from build123d import *

# Parameters (mm, degrees)
F0_R     = 17.275
F1_DEPTH = 18
F3_D     = 32
F4_R     = 16.275
F5_DEPTH = 5
F6_R     = 4.99999


# Not quite as in the source:
# - a fillet or chamfer is up to 0.001 mm smaller than in the source, because OpenCascade refuses the exact size


with BuildPart() as f1:
    # F0 (on Front) → F1 (new body)
    with BuildSketch(Plane.XZ):
        Circle(F0_R)
    extrude(amount=F1_DEPTH)

    # F3 (through all)
    with Locations(Plane(origin=(0, 0, 0), x_dir=(1, 0, 0), z_dir=(0, 1, 0))):
        with Locations((0, 0)):
            Hole(F3_D / 2)

    # F4 (on Front) → F5 (join)
    with BuildSketch(Plane.XZ):
        Circle(F4_R)
    extrude(amount=-F5_DEPTH)

    # F6 (radius 5 in the source; OpenCascade refuses exactly that, so slightly less here)
    f6_edges = [f1.edges().sort_by_distance(p)[0] for p in [
        (-16.275, 5, 0),
    ]]
    fillet(f6_edges, radius=F6_R)


solid = f1.part
Part model, mm, in its own coordinate system. A direction names the side the tool comes from. Coordinates: 2 decimals unless noted, no trailing zeros. Order: outer loops, then holes, each group sorted by start corner. A loop starts at its lowest first (then second) coordinate and runs counter-clockwise, first axis right, second up.
(1) Slice it at C-C, the plane y = -10.75. Write the cut outline in (x, z) (3 decimals), and give its area (3 significant figures).
Check sheet entries:
outline: circle Ø34.55 at (0, 0); hole circle Ø32 at (0, 0)
area: 133 mm2
(2) Pull direction Z, two halves, no side cores. Call faces 1 (the face through (15.958, -8.874, -6.616)), 2 (the face through (0, 0, 0)), 3 (the face through (11.44, -18, -11.44)): pulls with the +Z half, pulls with the -Z half, needs draft (parallel to the pull), parting line crosses it, or undercut.
Check sheet entries:
face 1: parting line crosses it
face 2: undercut
face 3: needs draft
(3) Tool access for faces 4 (the face through (0, 5, 0)), 5 (the face through (-12, 0, 12)), 6 (the face through (3.47, -9.13, 15.62)): list every direction of +Z, -Z, +X, -X, +Y, -Y with a clear straight run to the whole face (end or side of a thin tool).
Check sheet entries:
face 4: +Z, -Z, +X, -X, +Y
face 5: +Y
face 6: -Y
(4) Slice it at D-D, the plane y = 1. Write the cut outline in (x, z).
Check sheet entries:
outline: circle Ø32.35 at (0, 0)
(5) Pin check, flat tips, straight feed: pin 1 Ø16 at (x, z) = (-3.5, 7) entering from -Y; pin 2 Ø1.5 at (x, z) = (5, 13) entering from +Y; pin 3 Ø10 at (y, z) = (-7, -6) entering from +X. Stop position of each tip, or through.
Check sheet entries:
pin 1: stops at y = 0
pin 2: stops at y = 4.62
pin 3: stops at x = 17.25
(6) Probe L1, parallel to Z at x = 0, y = -3.75 (3 decimals); L2, parallel to X at y = -4.25, z = -0.5; L3, parallel to Y at x = -8, z = -8. List the from-to ranges inside material, lowest first.
Check sheet entries:
L1: z = -17.275 to -16, 16 to 17.275
L2: x = -17.27 to -15.99, 15.99 to 17.27
L3: y = 0 to 5
